from build123d import *

# Parameters (mm, degrees)
BOSS_EXTRUDE1_DEPTH            = 1.5
M3_CLEARANCE_HOLE1_D           = 3.4
M3_CLEARANCE_HOLE1_CSINK_D     = 3.45
M3_CLEARANCE_HOLE1_CSINK_ANGLE = 90


with BuildPart() as part:
    # Sketch1 → Boss-Extrude1 (new, symmetric)
    with BuildSketch(Plane(origin=(0, 0, 0), x_dir=(1, 0, 0), z_dir=(0, 1, 0))):
        Polygon((50, 15), (47, 15), (40.5, 15), (40.5, 12), (31.5, 12), (31.5, 15), (22.5, 15), (22.5, 12), (13.5, 12), (13.5, 15), (4.5, 15), (4.5, 12), (-4.5, 12), (-4.5, 15), (-13.5, 15), (-13.5, 12), (-22.5, 12), (-22.5, 15), (-31.5, 15), (-31.5, 12), (-40.5, 12), (-40.5, 15), (-47, 15), (-50, 15), (-50, 12), (-50, 4.5), (-47, 4.5), (-47, -4.5), (-50, -4.5), (-50, -12), (-50, -15), (-47, -15), (-40.5, -15), (-40.5, -12), (-31.5, -12), (-31.5, -15), (-22.5, -15), (-22.5, -12), (-13.5, -12), (-13.5, -15), (-4.5, -15), (-4.5, -12), (4.5, -12), (4.5, -15), (13.5, -15), (13.5, -12), (22.5, -12), (22.5, -15), (31.5, -15), (31.5, -12), (40.5, -12), (40.5, -15), (47, -15), (50, -15), (50, -12), (50, -4.5), (47, -4.5), (47, 4.5), (50, 4.5), (50, 12), align=None)
    extrude(amount=BOSS_EXTRUDE1_DEPTH, both=True)

    # M3 Clearance Hole1 (through all)
    with Locations(Plane(origin=(0, 1.5, 0), x_dir=(1, 0, 0), z_dir=(0, 1, 0))):
        with Locations((-30, -3), (30, -3)):
            CounterSinkHole(M3_CLEARANCE_HOLE1_D / 2, M3_CLEARANCE_HOLE1_CSINK_D / 2, counter_sink_angle=M3_CLEARANCE_HOLE1_CSINK_ANGLE)


solid = part.part
Geometry: final body of the model. Coordinates: model frame, mm. A direction names the side the tool comes from. Round coordinates to 2 decimals unless told otherwise and drop trailing zeros. Loops run counter-clockwise (first coordinate to the right, second up) from the corner with the lowest first, then second, coordinate; pieces in that order, holes last. Notation, with made-up numbers: M 86.5,89.5 L 120.5,89.5 A11 cw 120.5,106.5 Z; hole C -15,10.25 d7. An arc over 180 degrees is marked long. Put each result on its own line as item: value. Start each with the question number.
(1) Contact query for flat-ended pins moving along their axis: pin 1 Ø1.5 at (x, y) = (-34, 0.5) entering from -Z; pin 2 Ø1 at (x, y) = (34.5, -0.5) entering from +Z. Output: stop coordinate, or through.
(2) Section query B-B (x = -30). Return loops of the section in (y, z) (3 decimals), then the cut area to 3 significant figures.
(3) Draft query along X for faces 5 (the face through (-9, 0, 15)), 6 (the face through (-18, 0, 12)), 7 (the face through (50, 0, 10)). Return one class per face: +X half, -X half, draft (parallel to the pull), parting line (faces both ways), or undercut.
(4) Section query A-A (z = 3). Return loops of the section in (x, y) (3 decimals), then the cut area to 3 significant figures.
(5) Set-up query: faces 1 (the face through (31.5, 0, -13)), 2 (the face through (-48, 0, 4.5)), 3 (the face through (48, 0, -4.5)), 4 (the face through (4.5, 0, 13)). Return all of +Z, -Z, +X, -X, +Y, -Y with unobstructed straight access to the full face (end or side cutting, diameter ignored); none if empty.
(6) Section query D-D (y = 0.7). State how many separate pieces and enclosed holes the cut face has, then the cut area to 3 significant figures.
(7) Section query C-C (z = 13.25). Return loops of the section in (x, y).
(8) Material intervals for line 1 along X through (y, z) = (-0.35, -13.75); line 2 along Z through (x, y) = (-30, 0.7); line 3 along Z through (x, y) = (-29, 0.1), sorted ascending. Write a range as [from, to].
Findings below:
1. pin 1: stops at z = -12
1. pin 2: stops at z = 12
2. outline: M -1.5,-15 L 1.5,-15 L 1.5,1.275 L 1.475,1.3 L -1.5,1.3 Z; M -1.5,4.7 L 1.475,4.7 L 1.5,4.725 L 1.5,15 L -1.5,15 Z
2. area: 79.8 mm2
3. face 5: draft
3. face 6: undercut
3. face 7: +X half
4. outline: M -47,-1.5 L -31.7,-1.5 L -31.7,1.475 L -31.725,1.5 L -47,1.5 Z; M -28.3,-1.5 L 28.3,-1.5 L 28.3,1.475 L 28.275,1.5 L -28.275,1.5 L -28.3,1.475 Z; M 31.7,-1.5 L 47,-1.5 L 47,1.5 L 31.725,1.5 L 31.7,1.475 Z
4. area: 262 mm2
5. face 1: -Z, +Y, -Y
5. face 2: -X, +Y, -Y
5. face 3: +X, +Y, -Y
5. face 4: +Z, +Y, -Y
6. separate pieces: 1
6. enclosed holes: 2
6. area: 2,660 mm2
7. outline: M -50,-1.5 L -40.5,-1.5 L -40.5,1.5 L -50,1.5 Z; M -31.5,-1.5 L -22.5,-1.5 L -22.5,1.5 L -31.5,1.5 Z; M -13.5,-1.5 L -4.5,-1.5 L -4.5,1.5 L -13.5,1.5 Z; M 4.5,-1.5 L 13.5,-1.5 L 13.5,1.5 L 4.5,1.5 Z; M 22.5,-1.5 L 31.5,-1.5 L 31.5,1.5 L 22.5,1.5 Z; M 40.5,-1.5 L 50,-1.5 L 50,1.5 L 40.5,1.5 Z
8. line 1: x = [-50, -40.5], [-31.5, -22.5], [-13.5, -4.5], [4.5, 13.5], [22.5, 31.5], [40.5, 50]
8. line 2: z = [-15, 1.3], [4.7, 15]
8. line 3: z = [-15, 1.63], [4.37, 15]
